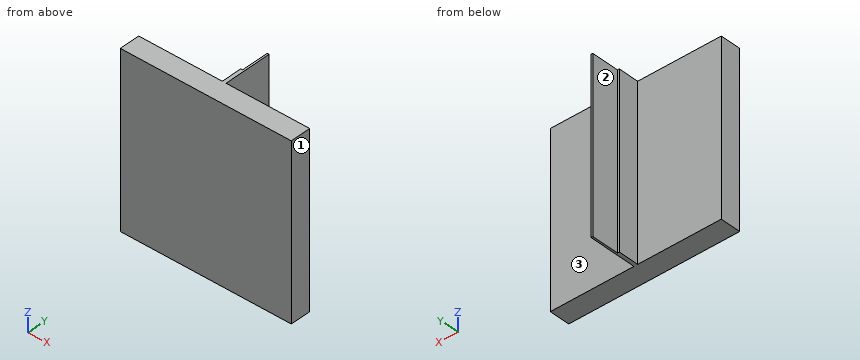
Autodesk Inventor part; units mm, degrees
ref_plane "YZ Plane" through (0, 0, 0) normal (1, 0, 0) x (0, 1, 0)
ref_plane "XZ Plane" through (0, 0, 0) normal (0, 1, 0) x (-1, 0, 0)
ref_plane "XY Plane" through (0, 0, 0) normal (0, 0, 1) x (1, 0, 0)
sketch "Sketch1" plane through (0, 0, 0) normal (0, 1, 0) x (-1, 0, 0)
  line L0 (0, 0) -> (-25, 0)
  line L1 (-25, 0) -> (-25, -25)
  line L2 (-25, -25) -> (0, -25)
  line L3 (0, -25) -> (0, 0)
  line L4 (-12.5, 0) -> (-12.5, -25)
  line L5 (-12.5, 0) -> (-12.772, 0)
  line L6 (-12.772, 0) -> (-12.772, -25)
  line L7 (-25, -25) -> (0, -25)
  line L8 (0, -25) -> (0, -26.7912)
  line L9 (0, -26.7912) -> (-25, -26.7912)
  line L10 (-25, -26.7912) -> (-25, -25)
  line L11 (-12.5, -26.7912) -> (-12.5, -25)
  line L12 (-12.228, 0) -> (-12.228, -25)
  dimension "d0" = 25
  dimension "d1" = 25
  dimension "d2" = 0.272
extrude "Extrusion1" add sketch "Sketch1" against normal blind 3 contours L3 L2 L12 L0 | L12 L2 L4 L0 | L4 L2 L6 L0 | L6 L2 L1 L0
extrude "Extrusion2" add sketch "Sketch1" along normal blind 7 contours L4 L2 L6 L0
extrude "Extrusion3" add sketch "Sketch1" along normal blind 3 contours L12 L2 L4 L0
sketch "Sketch2" plane through (25, -3, -25) normal (0, 0, -1) x (-1, 0, 0)
  line L0 (12.5, 6) -> (12.5, 10)
  line L1 (12.5, 10) -> (12.5, 30.188)
  point P0 (25, 3)
properties part number "podłoga"
The model under review builds one solid part; all positions refer to its coordinate system, in mm. Face numbers are marked on the shaded views. A direction names the side the tool comes from. Give positions to 0.01 mm unless a question says otherwise; leave off trailing zeros. Write each loop counter-clockwise with the first axis right and the second up, starting at its lowest first coordinate (ties: lowest second). Pieces come first, ordered by that corner, then holes.
1. Tool access review of the marked faces 1, 2 and 3: name each direction out of +Z, -Z, +X, -X, +Y, -Y from which nothing blocks a thin tool from reaching the whole face with its end or side.
2. Add section C-C, the plane x = 23.5. Write out the cut boundary in (y, z), plus the area to 3 significant figures.
3. Add section B-B, the plane y = 3.5. Write out the cut boundary in (x, z), plus the area to 3 significant figures.
4. Wall thickness on L1, parallel to X at y = 3.25, z = -17.5; L2, parallel to Y at x = 9.5, z = -10.25; L3, parallel to X at y = 1.75, z = -10.5: over which ranges is each line inside the solid? List them lowest first.
5. For P1, Ø6, axis at y = 5.5, z = -8.5, coming from the -X side; P2, Ø1, axis at x = 19, y = -0.5, coming from the +Z side; P3, Ø2, axis at y = 2, z = -8, coming from the +X side, all flat-tipped, find the tip position at first contact; note any pin that passes through.
6. Add section A-A, the plane z = -17.5. Write out the cut boundary in (x, y), plus the area to 3 significant figures.
Worked answers:
1. face 1: +Z, -Z, +X, +Y, -Y
1. face 2: +Z, -Z, -X, +Y
1. face 3: +Z, -Z, +X, +Y
2. outline: (-3, -25) - (0, -25) - (0, 0) - (-3, 0) - close
2. area: 75.0 mm2
3. outline: (12.5, -25) - (12.77, -25) - (12.77, 0) - (12.5, 0) - close
3. area: 6.80 mm2
4. L1: x = 12.5 to 12.77
4. L2: y = -3 to 0
4. L3: x = 12.23 to 12.77
5. P1: stops at x = 12.23
5. P2: stops at z = 0
5. P3: stops at x = 12.77
6. outline: (0, -3) - (25, -3) - (25, 0) - (12.77, 0) - (12.77, 7) - (12.5, 7) - (12.5, 3) - (12.23, 3) - (12.23, 0) - (0, 0) - close
6. area: 77.7 mm2
